```python
from build123d import *

# Parameters (mm, degrees)
SKETCH1_W           = 50.8
SKETCH1_H           = 50.8
SKETCH1_W_2         = 44.416753927
SKETCH1_H_2         = 44.416753927
BOSS_EXTRUDE1_DEPTH = 787.4
SKETCH2_R           = 6.35
CUT_EXTRUDE1_DEPTH  = 51.8
CUT_EXTRUDE2_DEPTH  = 76.2


with BuildPart() as part:
    # Sketch1 → Boss-Extrude1 (new body)
    with BuildSketch(Plane(origin=(0, 0, 0), x_dir=(1, 0, 0), z_dir=(0, 1, 0))):
        Rectangle(SKETCH1_W, SKETCH1_H)
        with Locations((-0.016623037, 0.016623037)):
            Rectangle(SKETCH1_W_2, SKETCH1_H_2, mode=Mode.SUBTRACT)
    extrude(amount=BOSS_EXTRUDE1_DEPTH)

    # Sketch2 → Cut-Extrude1 (cut, through all)
    with BuildSketch(Plane.ZY.offset(25.4)):
        with Locations((0, 50.8)):
            Circle(SKETCH2_R)
        with Locations((0, 177.8)):
            Circle(SKETCH2_R)
        with Locations((0, 609.6)):
            Circle(SKETCH2_R)
        with Locations((0, 736.6)):
            Circle(SKETCH2_R)
    extrude(amount=-CUT_EXTRUDE1_DEPTH, mode=Mode.SUBTRACT)

    # Sketch3 → Cut-Extrude2 (cut)
    with BuildSketch(Plane.ZY.offset(25.4)):
        with BuildLine():
            Line((-12.7, 210.943226022), (6.210922198, 200.025))
            ThreePointArc((6.210922198, 200.025), (12.560922198, 200.025), (15.735922198, 205.524261314))
            Line((15.735922198, 205.524261314), (15.735922198, 227.360713358))
            ThreePointArc((15.735922198, 227.360713358), (12.560922198, 232.859974672), (6.210922198, 232.859974672))
            Line((6.210922198, 232.859974672), (-12.7, 221.94174865))
            ThreePointArc((-12.7, 221.94174865), (-15.875, 216.442487336), (-12.7, 210.943226022))
        make_face()
        with BuildLine():
            Line((12.7, 264.382019928), (-6.35, 275.380542556))
            ThreePointArc((-6.35, 275.380542556), (-12.7, 275.380542556), (-15.875, 269.881281242))
            Line((-15.875, 269.881281242), (-15.875, 247.884235986))
            ThreePointArc((-15.875, 247.884235986), (-12.7, 242.384974672), (-6.35, 242.384974672))
            Line((-6.35, 242.384974672), (12.7, 253.3834973))
            ThreePointArc((12.7, 253.3834973), (15.875, 258.882758614), (12.7, 264.382019928))
        make_face()
        with BuildLine():
            Line((-12.7, 290.529340383), (6.210922198, 279.611114361))
            ThreePointArc((6.210922198, 279.611114361), (12.560922198, 279.611114361), (15.735922198, 285.110375675))
            Line((15.735922198, 285.110375675), (15.735922198, 306.946827719))
            ThreePointArc((15.735922198, 306.946827719), (12.560922198, 312.446089033), (6.210922198, 312.446089033))
            Line((6.210922198, 312.446089033), (-12.7, 301.527863011))
            ThreePointArc((-12.7, 301.527863011), (-15.875, 296.028601697), (-12.7, 290.529340383))
        make_face()
        with BuildLine():
            Line((12.7, 343.968134289), (-6.35, 354.966656917))
            ThreePointArc((-6.35, 354.966656917), (-12.7, 354.966656917), (-15.875, 349.467395603))
            Line((-15.875, 349.467395603), (-15.875, 327.470350347))
            ThreePointArc((-15.875, 327.470350347), (-12.7, 321.971089033), (-6.35, 321.971089033))
            Line((-6.35, 321.971089033), (12.7, 332.969611661))
            ThreePointArc((12.7, 332.969611661), (15.875, 338.468872975), (12.7, 343.968134289))
        make_face()
        with BuildLine():
            Line((-12.7, 370.115454744), (6.210922198, 359.197228722))
            ThreePointArc((6.210922198, 359.197228722), (12.560922198, 359.197228722), (15.735922198, 364.696490036))
            Line((15.735922198, 364.696490036), (15.735922198, 386.53294208))
            ThreePointArc((15.735922198, 386.53294208), (12.560922198, 392.032203394), (6.210922198, 392.032203394))
            Line((6.210922198, 392.032203394), (-12.7, 381.113977372))
            ThreePointArc((-12.7, 381.113977372), (-15.875, 375.614716058), (-12.7, 370.115454744))
        make_face()
        with BuildLine():
            Line((12.7, 423.55424865), (-6.35, 434.552771278))
            ThreePointArc((-6.35, 434.552771278), (-12.7, 434.552771278), (-15.875, 429.053509964))
            Line((-15.875, 429.053509964), (-15.875, 407.056464708))
            ThreePointArc((-15.875, 407.056464708), (-12.7, 401.557203394), (-6.35, 401.557203394))
            Line((-6.35, 401.557203394), (12.7, 412.555726022))
            ThreePointArc((12.7, 412.555726022), (15.875, 418.054987336), (12.7, 423.55424865))
        make_face()
        with BuildLine():
            Line((-12.7, 449.701569105), (6.210922198, 438.783343083))
            ThreePointArc((6.210922198, 438.783343083), (12.560922198, 438.783343083), (15.735922198, 444.282604397))
            Line((15.735922198, 444.282604397), (15.735922198, 466.119056441))
            ThreePointArc((15.735922198, 466.119056441), (12.560922198, 471.618317755), (6.210922198, 471.618317755))
            Line((6.210922198, 471.618317755), (-12.7, 460.700091733))
            ThreePointArc((-12.7, 460.700091733), (-15.875, 455.200830419), (-12.7, 449.701569105))
        make_face()
        with BuildLine():
            Line((12.7, 503.140363011), (-6.35, 514.138885639))
            ThreePointArc((-6.35, 514.138885639), (-12.7, 514.138885639), (-15.875, 508.639624325))
            Line((-15.875, 508.639624325), (-15.875, 486.642579069))
            ThreePointArc((-15.875, 486.642579069), (-12.7, 481.143317755), (-6.35, 481.143317755))
            Line((-6.35, 481.143317755), (12.7, 492.141840383))
            ThreePointArc((12.7, 492.141840383), (15.875, 497.641101697), (12.7, 503.140363011))
        make_face()
        with BuildLine():
            Line((-12.7, 529.287683466), (6.210922198, 518.369457444))
            ThreePointArc((6.210922198, 518.369457444), (12.560922198, 518.369457444), (15.735922198, 523.868718758))
            Line((15.735922198, 523.868718758), (15.735922198, 545.705170802))
            ThreePointArc((15.735922198, 545.705170802), (12.560922198, 551.204432116), (6.210922198, 551.204432116))
            Line((6.210922198, 551.204432116), (-12.7, 540.286206094))
            ThreePointArc((-12.7, 540.286206094), (-15.875, 534.78694478), (-12.7, 529.287683466))
        make_face()
        with BuildLine():
            Line((12.7, 582.726477372), (-6.35, 593.725))
            ThreePointArc((-6.35, 593.725), (-12.7, 593.725), (-15.875, 588.225738686))
            Line((-15.875, 588.225738686), (-15.875, 566.22869343))
            ThreePointArc((-15.875, 566.22869343), (-12.7, 560.729432116), (-6.35, 560.729432116))
            Line((-6.35, 560.729432116), (12.7, 571.727954744))
            ThreePointArc((12.7, 571.727954744), (15.875, 577.227216058), (12.7, 582.726477372))
        make_face()
    extrude(amount=-CUT_EXTRUDE2_DEPTH, mode=Mode.SUBTRACT)


solid = part.part
```
Check sheet for the modelled part. Datum: model origin and axes. Units: mm. A direction names the side the tool comes from. Give positions to 0.01 mm unless a question says otherwise; leave off trailing zeros. Loops run counter-clockwise (first coordinate to the right, second up) from the corner with the lowest first, then second, coordinate; pieces in that order, holes last. Notation, with made-up numbers: (81, -5) - (135, -5) arc R9 ccw to (135, 8) - close; hole circle Ø10 at (-30.5, 37). An arc over 180 degrees is marked (long way). One line per question, with ' | ' between items. Start each with the question number.
1. Draft check along Z on faces 1 (the flat face through (0, 787.4, -23)), 2 (the flat face through (0, 388, -22.225)), 3 (the flat face through (0, 388, -25.4)), 4 (the cylindrical face through (-23.83, 730.4, -1.38)). Enter one of: released by +Z, released by -Z, zero draft, split by the parting line, or undercut.
2. Cross-section at B-B, the plane x = -6. Enter the section's corners in (y, z) (3 decimals), plus the area to 3 significant figures.
3. Gauge pin test, flat ends, axial feed: pin 1 Ø13.5 at (y, z) = (215.5, -8) entering from +X; pin 2 Ø11.5 at (y, z) = (736.6, 0) entering from +X. Record the tip position at first contact, or that the pin passes through.
4. Cross-section at A-A, the plane y = 177.8. Enter the section's corners in (x, z) (3 decimals).
5. Material ranges on line 1 along X through (y, z) = (516, -7) (3 decimals); line 2 along Z through (x, y) = (24, 736), recorded low to high. Write a range as [from, to].
6. Set-up check for faces 5 (the flat face through (-22.225, 388, -5)), 6 (the cylindrical face through (23.77, 603.4, -1.38)): record each of +Z, -Z, +X, -X, +Y, -Y from which the full face is reachable in a straight line by a thin tool's end or side.
Check result:
1) face 1: zero draft | face 2: undercut | face 3: released by -Z | face 4: undercut
2) outline: (0, -25.4) - (787.4, -25.4) - (787.4, -22.225) - (0, -22.225) - close; (0, 22.192) - (787.4, 22.192) - (787.4, 25.4) - (0, 25.4) - close | area: 5,030 mm2
3) pin 1: stops at x = 25.4 | pin 2: passes through
4) outline: (-25.4, -25.4) - (25.4, -25.4) - (25.4, -6.35) - (22.192, -6.35) - (22.192, -22.225) - (-22.225, -22.225) - (-22.225, -6.35) - (-25.4, -6.35) - close; (-25.4, 6.35) - (-22.225, 6.35) - (-22.225, 22.192) - (22.192, 22.192) - (22.192, 6.35) - (25.4, 6.35) - (25.4, 25.4) - (-25.4, 25.4) - close
5) line 1: x = [-25.4, -22.225], [22.192, 25.4] | line 2: z = [-25.4, -6.32], [6.32, 25.4]
6) face 5: +Y, -Y | face 6: +X, -X
